Answer from the drawing. Dimensions are ordinates in mm from the lowest x, y and z of the part. Coordinates: 2 decimals unless noted, no trailing zeros. Write each loop counter-clockwise with the first axis right and the second up, starting at its lowest first coordinate (ties: lowest second). Pieces come first, ordered by that corner, then holes. Notation, with made-up numbers: (-25, -28) - (0, -28) arc R14 cw to (0, -11) - close; hole circle Ø9 at (-11.75, 84.5). An arc over 180 degrees is marked (long way). Use one line per item in the form item = value. Start each with the question number.
Item 1: A cutting plane is placed at D-D (x = 61.5). Write down the section's boundary in (y, z).
Item 2: A cutting plane is placed at A-A (y = 40). Write down the section's boundary in (x, z) (1 decimal).
Item 3: Given pin 1 (5 mm diameter, centred on x = 43.5, y = 51, fed in from -Z); pin 2 (1.8 mm diameter, centred on y = 37.5, z = 3, fed in from -X); pin 3 (3 mm diameter, centred on x = 81.86, y = 40, fed in from +Z), each flat-ended and moving along its own axis, determine where each tip first touches the part or whether it passes through.
Item 4: Consider probe 1 along Y at (x, z) = (4, 2.1); probe 2 along X at (y, z) = (5.5, 2.75) (1 decimal); probe 3 along Y at (x, z) = (61.5, 3.05). Determine where each line is inside the solid, lowest interval first.
Item 5: A cutting plane is placed at C-C (y = 29.5). Write down the section's boundary in (x, z) (1 decimal), then the cut area to 3 significant figures.
Item 6: A cutting plane is placed at B-B (z = 4). Write down the section's boundary in (x, y) (1 decimal).
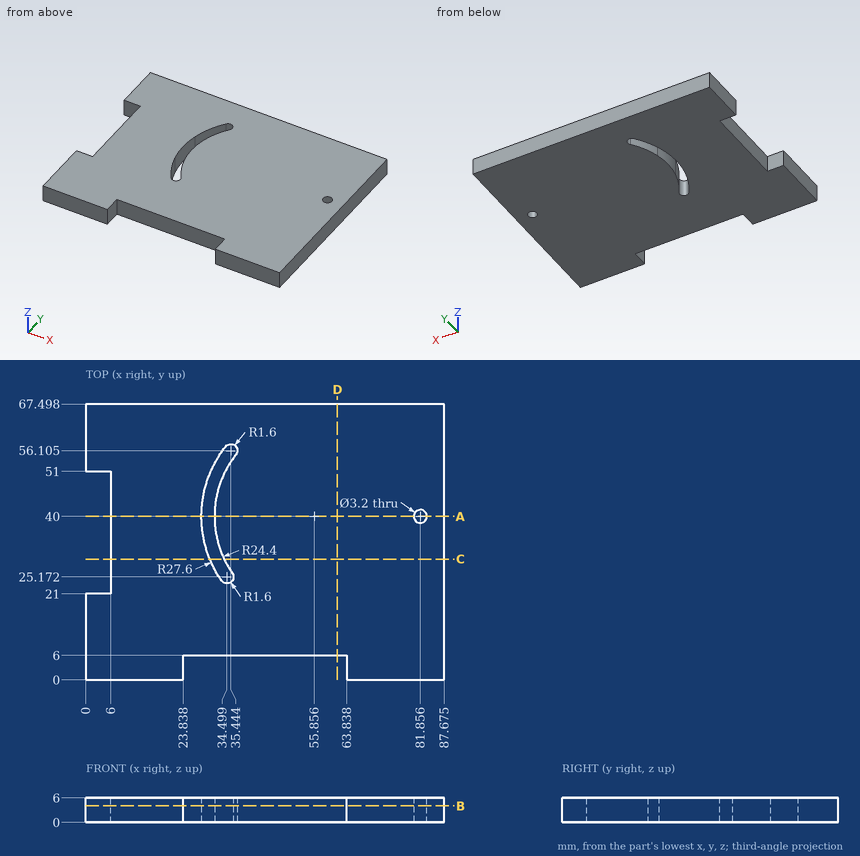
Answer:
q1.outline = (6, 0) - (67.5, 0) - (67.5, 6) - (6, 6) - close
q2.outline = (6, 0) - (28.3, 0) - (28.3, 6) - (6, 6) - close; (31.5, 0) - (80.3, 0) - (80.3, 6) - (31.5, 6) - close; (83.5, 0) - (87.7, 0) - (87.7, 6) - (83.5, 6) - close
q3.pin_1 = 0
q3.pin_2 = 6
q3.pin_3 = through
q4.probe_1 = 0 to 21, 51 to 67.5
q4.probe_2 = 0 to 23.8, 63.8 to 87.7
q4.probe_3 = 6 to 67.5
q5.outline = (6, 0) - (30.3, 0) - (30.3, 6) - (6, 6) - close; (33.8, 0) - (87.7, 0) - (87.7, 6) - (33.8, 6) - close
q5.area = 469 mm²
q6.outline = (0, 0) - (23.8, 0) - (23.8, 6) - (63.8, 6) - (63.8, 0) - (87.7, 0) - (87.7, 67.5) - (0, 67.5) - (0, 51) - (6, 51) - (6, 21) - (0, 21) - close; hole (33.2, 24.3) arc R1.6 ccw to (35.8, 26.1) arc R24.4 cw to (36.7, 55.1) arc R1.6 ccw to (34.2, 57.1) arc R27.6 ccw to start; hole circle Ø3.2 at (81.9, 40)
